Here's how the part is built. I have some questions about the finished solid (model axes, mm). Face numbers are marked on the shaded views. A direction names the side the tool comes from. Give positions to 0.01 mm unless a question says otherwise; leave off trailing zeros. Loops run counter-clockwise (first coordinate to the right, second up) from the corner with the lowest first, then second, coordinate; pieces in that order, holes last.
Q1. If we section it at B-B (y = 47): Please give me the cut outline in (x, z) (3 decimals).
Q2. We'd pull the mould along X, two halves only. Please class the marked faces 3, 4, 5 and 6: +X half, -X half, draft (parallel to the pull), parting line (faces both ways), or undercut.
Q3. I need wall thicknesses on line 1 (Y direction, x = 0, z = 11.7) (3 decimals); line 2 (Z direction, x = 6, y = 15.5) (3 decimals). Which ranges of each line are inside material? Lowest first, please.
Q4. If we section it at C-C (z = 2): Please give me the cut outline in (x, y) (3 decimals).
Q5. If we section it at A-A (x = 0): Please give me the cut outline in (y, z) (3 decimals).
Q6. For the marked faces 1 and 2, which set-ups out of +Z, -Z, +X, -X, +Y, -Y let a thin tool reach every point of the face, with its end or its side?
from build123d import *

# Parameters (mm, degrees)
SKETCH1_W               = 25.4
SKETCH1_H               = 25.4
SKETCH1_W_2             = 19.05
SKETCH1_H_2             = 19.05
BOSS_EXTRUDE1_DEPTH     = 1219.2
FILLET1_R               = 2.1082
SKETCH2_OUTSIDE_W       = 271.346
SKETCH2_OUTSIDE_H       = 1465.146
SKETCH2_OUTSIDE_W_2     = 161.404490431
SKETCH2_OUTSIDE_H_2     = 228.6
CUT_EXTRUDE1_DEPTH      = 1220.530684321
CUT_EXTRUDE3_DEPTH      = 231.35713577
CUT_EXTRUDE3_DEPTH_BACK = 231.35713577
SKETCH5_R               = 3.175


with BuildPart() as part:
    # Sketch1 → Boss-Extrude1 (new body)
    with BuildSketch(Plane(origin=(0, 0, 0), x_dir=(1, 0, 0), z_dir=(0, 1, 0))):
        Rectangle(SKETCH1_W, SKETCH1_H)
        Rectangle(SKETCH1_W_2, SKETCH1_H_2, mode=Mode.SUBTRACT)
    extrude(amount=BOSS_EXTRUDE1_DEPTH)

    # Fillet1
    fillet1_edges = [part.edges().sort_by_distance(p)[0] for p in [
        (9.525, 609.6, 9.525),
        (9.525, 609.6, -9.525),
        (-9.525, 609.6, -9.525),
        (-9.525, 609.6, 9.525),
        (-12.7, 609.6, -12.7),
        (12.7, 609.6, -12.7),
        (12.7, 609.6, 12.7),
        (-12.7, 609.6, 12.7),
    ]]
    fillet(fillet1_edges, radius=FILLET1_R)

    # Sketch2 outside → Cut-Extrude1 (cut, through all)
    with BuildSketch(Plane(origin=(12.7, 0, 0), x_dir=(0, 0, -1), z_dir=(1, 0, 0))):
        with Locations((0, 609.6)):
            Rectangle(SKETCH2_OUTSIDE_W, SKETCH2_OUTSIDE_H)
        with Locations((42.327264621, 114.3)):
            Rectangle(SKETCH2_OUTSIDE_W_2, SKETCH2_OUTSIDE_H_2, mode=Mode.SUBTRACT)
    extrude(amount=-CUT_EXTRUDE1_DEPTH, mode=Mode.SUBTRACT)

    # Sketch5 → Cut-Extrude3 (cut, two sides: drawn at the far end of the back side and taken through both)
    with BuildSketch(Plane.XY.offset(12.7).offset(-CUT_EXTRUDE3_DEPTH_BACK)):
        with Locations((0, 12.7)):
            Circle(SKETCH5_R)
        with Locations((0, 38.1)):
            Circle(SKETCH5_R)
    extrude(amount=CUT_EXTRUDE3_DEPTH + CUT_EXTRUDE3_DEPTH_BACK, mode=Mode.SUBTRACT)


solid = part.part
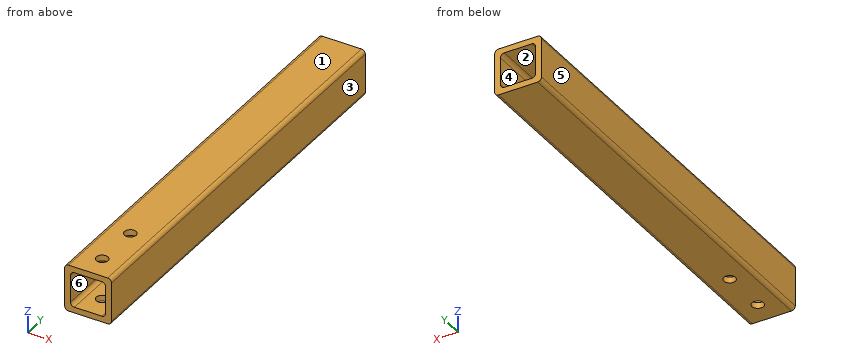
Check sheet entries:
1. outline: (-12.7, -10.592) arc R2.108 ccw to (-10.592, -12.7) - (10.592, -12.7) arc R2.108 ccw to (12.7, -10.592) - (12.7, 10.592) arc R2.108 ccw to (10.592, 12.7) - (-10.592, 12.7) arc R2.108 ccw to (-12.7, 10.592) - close; hole (-9.525, -7.417) arc R2.108 ccw to (-7.417, -9.525) - (7.417, -9.525) arc R2.108 ccw to (9.525, -7.417) - (9.525, 7.417) arc R2.108 ccw to (7.417, 9.525) - (-7.417, 9.525) arc R2.108 ccw to (-9.525, 7.417) - close
2. face 3: +X half
2. face 4: undercut
2. face 5: -X half
2. face 6: undercut
3. line 1: y = 0 to 9.525, 15.875 to 34.925, 41.275 to 228.6
3. line 2: z = -12.7 to -9.525, 9.525 to 12.7
4. outline: (-12.7, 0) - (-9.525, 0) - (-9.525, 228.6) - (-12.7, 228.6) - close; (9.525, 0) - (12.7, 0) - (12.7, 228.6) - (9.525, 228.6) - close
5. outline: (0, -12.7) - (9.525, -12.7) - (9.525, -9.525) - (0, -9.525) - close; (0, 9.525) - (9.525, 9.525) - (9.525, 12.7) - (0, 12.7) - close; (15.875, -12.7) - (34.925, -12.7) - (34.925, -9.525) - (15.875, -9.525) - close; (15.875, 9.525) - (34.925, 9.525) - (34.925, 12.7) - (15.875, 12.7) - close; (41.275, -12.7) - (228.6, -12.7) - (228.6, -9.525) - (41.275, -9.525) - close; (41.275, 9.525) - (228.6, 9.525) - (228.6, 12.7) - (41.275, 12.7) - close
6. face 1: +Z, +X, -X, +Y, -Y
6. face 2: +Y, -Y
